Design review of the part built by this model. Coordinates are the model's own, in mm. A direction names the side the tool comes from. Give positions to 0.01 mm unless a question says otherwise; leave off trailing zeros. Write each loop counter-clockwise with the first axis right and the second up, starting at its lowest first coordinate (ties: lowest second). Pieces come first, ordered by that corner, then holes. Notation, with made-up numbers: M 8.5,30.5 L 60.5,30.5 A27 cw 60.5,68.5 Z; hole C 78.5,-11 d5. An arc over 180 degrees is marked long. One line per item, written item: value. Start each with the question number.
```python
from build123d import *

# Parameters (mm, degrees)
SKETCH1_R           = 5
SKETCH1_R_2         = 1.05
SKETCH1_R_3         = 1.55
BOSS_EXTRUDE1_DEPTH = 2


with BuildPart() as part:
    # Sketch1 → Boss-Extrude1 (new body)
    with BuildSketch(Plane(origin=(0, 0, 0), x_dir=(1, 0, 0), z_dir=(0, 1, 0))):
        with BuildLine():
            Line((-2.668728536, 14.760687247), (-29, 10))
            Line((-29, 10), (-29, -10))
            Line((-29, -10), (-2.668728536, -14.760687247))
            ThreePointArc((-2.668728536, -14.760687247), (0, -15), (2.668728536, -14.760687247))
            Line((2.668728536, -14.760687247), (29, -10))
            Line((29, -10), (29, 10))
            Line((29, 10), (2.668728536, 14.760687247))
            ThreePointArc((2.668728536, 14.760687247), (0, 15), (-2.668728536, 14.760687247))
        make_face()
        with Locations(Location((0, 0, 0), (0, 0, 270))):
            Circle(SKETCH1_R, mode=Mode.SUBTRACT)
        with Locations(Location((-27, 0, 0), (0, 0, 270))):
            Circle(SKETCH1_R_2, mode=Mode.SUBTRACT)
        with Locations(Location((27, 0, 0), (0, 0, 270))):
            Circle(SKETCH1_R_2, mode=Mode.SUBTRACT)
        with Locations(Location((8.838834765, 8.838834765, 0), (0, 0, 270))):
            Circle(SKETCH1_R_3, mode=Mode.SUBTRACT)
        with Locations(Location((8.838834765, -8.838834765, 0), (0, 0, 270))):
            Circle(SKETCH1_R_3, mode=Mode.SUBTRACT)
        with Locations(Location((-8.838834765, -8.838834765, 0), (0, 0, 270))):
            Circle(SKETCH1_R_3, mode=Mode.SUBTRACT)
        with Locations(Location((-8.838834765, 8.838834765, 0), (0, 0, 270))):
            Circle(SKETCH1_R_3, mode=Mode.SUBTRACT)
        with BuildLine():
            Line((-20.728140636, -4.5), (-20.728140636, 4.5))
            ThreePointArc((-20.728140636, 4.5), (-18.728140636, 6.5), (-16.728140636, 4.5))
            Line((-16.728140636, 4.5), (-16.728140636, -4.5))
            ThreePointArc((-16.728140636, -4.5), (-18.728140636, -6.5), (-20.728140636, -4.5))
        make_face(mode=Mode.SUBTRACT)
    extrude(amount=BOSS_EXTRUDE1_DEPTH)


solid = part.part
```
Q1. Take a section at B-B, the plane z = 0. Give the boundary of the cut face in (x, y).
Q2. Take a section at D-D, the plane x = 8. Give the boundary of the cut face in (y, z), then the cut area to 3 significant figures.
Q3. Wall thickness on line 1 (X direction, y = 1, z = -9); line 2 (X direction, y = 0.8, z = 7.5); line 3 (Z direction, x = -9, y = 0.8): over which ranges is each line inside the solid? List them lowest first. Write a range as from..to.
Q4. The part is to be moulded in two halves that separate along Z. For faces 3 (the face through (15.65, 0.986, 12.414)), 4 (the face through (0, 1, -15)), 5 (the face through (-20.728, 1, 0)), 6 (the face through (-28.025, 0.986, -0.228)), say which applies: pulls with the +Z half, pulls with the -Z half, needs draft (parallel to the pull), parting line crosses it, or undercut.
Q5. Take a section at A-A, the plane x = 0. Give the boundary of the cut face in (y, z), then the cut area to 3 significant figures.
Q6. Machinability: for faces 1 (the face through (-16.728, 1, 0)), 2 (the face through (16.019, 0.986, -12.347)), which of the approach directions +Z, -Z, +X, -X, +Y, -Y give a long, thin tool a straight path to every point of the face, cutting with its end or side? Answer none if there is none.
Q7. Take a section at C-C, the plane z = -3. Give the boundary of the cut face in (x, y).
Results list:
1. outline: M -29,0 L -28.05,0 L -28.05,2 L -29,2 Z; M -25.95,0 L -20.73,0 L -20.73,2 L -25.95,2 Z; M -16.73,0 L -5,0 L -5,2 L -16.73,2 Z; M 5,0 L 25.95,0 L 25.95,2 L 5,2 Z; M 28.05,0 L 29,0 L 29,2 L 28.05,2 Z
2. outline: M 0,-13.8 L 2,-13.8 L 2,-10.14 L 0,-10.14 Z; M 0,-7.54 L 2,-7.54 L 2,7.54 L 0,7.54 Z; M 0,10.14 L 2,10.14 L 2,13.8 L 0,13.8 Z
2. area: 44.8 mm^2
3. line 1: x = -29..-10.38, -7.3..7.3, 10.38..29
3. line 2: x = -29..-9.62, -8.06..8.06, 9.62..29
3. line 3: z = -13.62..-10.38, -7.3..7.3, 10.38..13.62
4. face 3: pulls with the +Z half
4. face 4: pulls with the -Z half
4. face 5: undercut
4. face 6: undercut
5. outline: M 0,-15 L 2,-15 L 2,-5 L 0,-5 Z; M 0,5 L 2,5 L 2,15 L 0,15 Z
5. area: 40.0 mm^2
6. face 1: +Y, -Y
6. face 2: -Z, +X, +Y, -Y
7. outline: M -29,0 L -20.73,0 L -20.73,2 L -29,2 Z; M -16.73,0 L -4,0 L -4,2 L -16.73,2 Z; M 4,0 L 29,0 L 29,2 L 4,2 Z
